The model under review builds one solid part; all positions refer to its coordinate system, in mm. Face numbers are marked on the shaded views. A direction names the side the tool comes from. Give positions to 0.01 mm unless a question says otherwise; leave off trailing zeros. Order: outer loops, then holes, each group sorted by start corner. A loop starts at its lowest first (then second) coordinate and runs counter-clockwise, first axis right, second up. Notation, with made-up numbers: M -34,-15 L -12,-15 A20 cw -12,-4 Z; hole C 15.5,33.25 d9. An arc over 180 degrees is marked long. One line per question, with ' | ' between items. Start each with the question number.
1. Wall thickness on L1, parallel to X at y = -8.2, z = 23.2; L2, parallel to Z at x = -29, y = -7.4; L3, parallel to X at y = -7, z = 22.5: over which ranges is each line inside the solid? List them lowest first.
2. For the marked faces 5, 6, 7 and 8, list the 3-axis set-ups (+Z, -Z, +X, -X, +Y, -Y) from which the entire face can be reached by the end or side of a thin tool; tool diameter is ignored.
3. We need section A-A on x = -29. Write out the cut boundary in (y, z).
4. The part is to be moulded in two halves that separate along X. For the marked faces 1, 2, 3 and 4, say which applies: +X half, -X half, draft (parallel to the pull), parting line (faces both ways), or undercut.
5. We need section C-C on x = -7.5. Write out the cut boundary in (y, z).
6. We need section B-B on z = 10.5. Write out the cut boundary in (x, y).
7. Insertion check: P1, Ø1.3, axis at x = -56.5, y = 4.5, coming from the +Z side; P2, Ø6, axis at x = 21, z = 29, coming from the +Y side; P3, Ø5, axis at y = 5, z = 9.5, coming from the +X side. Each pin has a flat end and moves straight along its axis. Give the tip position at first contact, or say it passes through.
```python
from build123d import *

# Parameters (mm, degrees)
F2_DEPTH     = 9
F3_DEPTH     = 10
F4_R         = 4.1
F4_R_2       = 2.5
F4_R_3       = 1.6
F5_DEPTH     = 24.8
F6_DEPTH     = 3
F4_R_4       = 5
F7_DEPTH     = 6
F4_R_5       = 7.75
F8_DEPTH     = 5
F9_R         = 1.75
F10_DEPTH    = 158.2
F9_R_2       = 3.25
F11_DEPTH    = 2.4
F12_R        = 3.25
F13_DEPTH    = 2.4
F14_R        = 3.4
F14_R_2      = 1.75
F15_DEPTH    = 3
F16_DEPTH    = 25
F17_W        = 100
F17_H        = 9
F18_DEPTH    = 1.1
F20_START    = -1.4
F19_R        = 1.75
F20_DEPTH    = 2.6
F21_DEPTH    = 4.2
F22_W        = 6.7549981495
F22_H        = 2.6
F23_DEPTH    = 4.5
F24_W        = 19
F24_H        = 10
F25_DEPTH    = 16
F26_SIZE     = 5
F27_W        = 19
F27_H        = 10
F28_DEPTH    = 16
F29_SIZE     = 5
F30_R        = 3.15
F31_DEPTH    = 25
F32_R        = 0.4
F33_W        = 87.1225009252
F33_H        = 9
F34_DEPTH    = 4
F35_T1_DEPTH = 9
F37_DEPTH    = 4


# Not quite as in the source:
# - a fillet or chamfer that OpenCascade refuses, or shapes differently, is made with other operations: its cross-section is extruded or revolved along the edge and cut away or added


with BuildPart() as f2:
    # F1 (on face) → F2 (new body)
    with BuildSketch(Plane.XZ):
        Polygon((-55, 28), (-64, 28), (-64, -6), (0, -6), (64, -6), (64, 28), (55, 28), (55, 32.2), (0, 32.2), (-55, 32.2), align=None)
    extrude(amount=F2_DEPTH)

    # F0 (on Front) → F3 (join)
    with BuildSketch(Plane.XZ):
        with BuildLine():
            Line((-57.5, 28), (-64, 28))
            Line((-64, 28), (-64, -6))
            Line((-64, -6), (-43.5, -6))
            Line((-43.5, -6), (-43.5, 0))
            Line((-43.5, 0), (-55, 0))
            ThreePointArc((-55, 0), (-55.3535533906, -0.1464466094), (-55.5, -0.5))
            Line((-55.5, -0.5), (-55.5, -1.5))
            Line((-55.5, -1.5), (-59, -1.5))
            Line((-59, -1.5), (-59, 6.5))
            Line((-59, 6.5), (-54.7, 6.5))
            ThreePointArc((-54.7, 6.5), (-54.3464466094, 6.6464466094), (-54.2, 7))
            Line((-54.2, 7), (-54.2, 13.5))
            ThreePointArc((-54.2, 13.5), (-54.3464466094, 13.8535533906), (-54.7, 14))
            Line((-54.7, 14), (-59, 14))
            Line((-59, 14), (-59, 20.5))
            Line((-59, 20.5), (-57.5, 20.5))
            ThreePointArc((-57.5, 20.5), (-57.1464466094, 20.6464466094), (-57, 21))
            Line((-57, 21), (-57, 27.5))
            ThreePointArc((-57, 27.5), (-57.1464466094, 27.8535533906), (-57.5, 28))
        make_face()
        with BuildLine():
            Line((43.5, -6), (64, -6))
            Line((64, -6), (64, 28))
            Line((64, 28), (57.5, 28))
            ThreePointArc((57.5, 28), (57.1464466094, 27.8535533906), (57, 27.5))
            Line((57, 27.5), (57, 21))
            ThreePointArc((57, 21), (57.1464466094, 20.6464466094), (57.5, 20.5))
            Line((57.5, 20.5), (59, 20.5))
            Line((59, 20.5), (59, 14))
            Line((59, 14), (54.7, 14))
            ThreePointArc((54.7, 14), (54.3464466094, 13.8535533906), (54.2, 13.5))
            Line((54.2, 13.5), (54.2, 7))
            ThreePointArc((54.2, 7), (54.3464466094, 6.6464466094), (54.7, 6.5))
            Line((54.7, 6.5), (59, 6.5))
            Line((59, 6.5), (59, -1.5))
            Line((59, -1.5), (55.5, -1.5))
            Line((55.5, -1.5), (55.5, -0.5))
            ThreePointArc((55.5, -0.5), (55.3535533906, -0.1464466094), (55, 0))
            Line((55, 0), (43.5, 0))
            Line((43.5, 0), (43.5, -6))
        make_face()
    extrude(amount=-F3_DEPTH)

    # F4 (on Front) → F5 (cut)
    with BuildSketch(Plane.XZ):
        with Locations((-29, 23.2)):
            Circle(F4_R)
        with Locations((-45, 23.2)):
            Circle(F4_R)
        with Locations((35.2, 26.5)):
            Circle(F4_R_2)
        with Locations((17.2, 26.5)):
            Circle(F4_R_2)
        with Locations((5.4, 20.2)):
            Circle(F4_R_3)
        with Locations((47, 20.2)):
            Circle(F4_R_3)
    extrude(amount=F5_DEPTH, mode=Mode.SUBTRACT)

    # F4 (on Front) → F6 (cut)
    with BuildSketch(Plane.XZ):
        Polygon((3.7112504626, 17.275), (7.0887495374, 17.275), (8.7774990748, 20.2), (7.0887495374, 23.125), (3.7112504626, 23.125), (2.0225009252, 20.2), align=None)
        with Locations((5.4, 20.2)):
            Circle(F4_R_3, mode=Mode.SUBTRACT)
        Polygon((45.3112504626, 17.275), (48.6887495374, 17.275), (50.3774990748, 20.2), (48.6887495374, 23.125), (45.3112504626, 23.125), (43.6225009252, 20.2), align=None)
        with Locations((47, 20.2)):
            Circle(F4_R_3, mode=Mode.SUBTRACT)
    extrude(amount=F6_DEPTH, mode=Mode.SUBTRACT)

    # F4 (on Front) → F7 (cut)
    with BuildSketch(Plane.XZ):
        with Locations((-45, 23.2)):
            Circle(F4_R_4)
        with Locations((-45, 23.2)):
            Circle(F4_R, mode=Mode.SUBTRACT)
        with Locations((-29, 23.2)):
            Circle(F4_R_4)
        with Locations((-29, 23.2)):
            Circle(F4_R, mode=Mode.SUBTRACT)
    extrude(amount=F7_DEPTH, mode=Mode.SUBTRACT)

    # F4 (on Front) → F8 (cut)
    with BuildSketch(Plane.XZ):
        with Locations((-29, 23.2)):
            Circle(F4_R_5)
        with Locations((-29, 23.2)):
            Circle(F4_R_4, mode=Mode.SUBTRACT)
        with Locations((-45, 23.2)):
            Circle(F4_R_5)
        with Locations((-45, 23.2)):
            Circle(F4_R_4, mode=Mode.SUBTRACT)
    extrude(amount=F8_DEPTH, mode=Mode.SUBTRACT)

    # F9 (on face) → F10 (cut)
    with BuildSketch(Plane(origin=(-64, 0, 0), x_dir=(0, -1, 0), z_dir=(-1, 0, 0))):
        with Locations((-5.2, 24.2)):
            Circle(F9_R)
    extrude(amount=-F10_DEPTH, mode=Mode.SUBTRACT)

    # F9 (on face) → F11 (cut)
    with BuildSketch(Plane(origin=(-64, 0, 0), x_dir=(0, -1, 0), z_dir=(-1, 0, 0))):
        with Locations((-5.2, 24.2)):
            Circle(F9_R_2)
        with Locations((-5.2, 24.2)):
            Circle(F9_R, mode=Mode.SUBTRACT)
    extrude(amount=-F11_DEPTH, mode=Mode.SUBTRACT)

    # F12 (on face) → F13 (cut)
    with BuildSketch(Plane.YZ.offset(64)):
        with Locations((5.2, 24.2)):
            Circle(F12_R)
    extrude(amount=-F13_DEPTH, mode=Mode.SUBTRACT)

    # F14 (on face) → F15 (cut)
    with BuildSketch(Plane(origin=(0, 0, -6), x_dir=(1, 0, 0), z_dir=(0, 0, -1))):
        with Locations((49.8, -5.1)):
            Circle(F14_R)
        with Locations((49.8, -5.1)):
            Circle(F14_R_2, mode=Mode.SUBTRACT)
        with Locations((-48.5, -5.1)):
            Circle(F14_R)
        with Locations((-48.5, -5.1)):
            Circle(F14_R_2, mode=Mode.SUBTRACT)
        with Locations((49.8, -5.1)):
            Circle(F14_R_2)
    extrude(amount=-F15_DEPTH, mode=Mode.SUBTRACT)

    # F14 (on face) → F16 (cut)
    with BuildSketch(Plane(origin=(0, 0, -6), x_dir=(1, 0, 0), z_dir=(0, 0, -1))):
        with Locations((49.8, -5.1)):
            Circle(F14_R_2)
        with Locations((-48.5, -5.1)):
            Circle(F14_R_2)
    extrude(amount=-F16_DEPTH, mode=Mode.SUBTRACT)

    # F17 (on face) → F18 (join)
    with BuildSketch(Plane.XY.offset(32.2)):
        with Locations((5, -4.5)):
            Rectangle(F17_W, F17_H)
    extrude(amount=F18_DEPTH)

    # F19 (on face) → F20 (cut)
    with BuildSketch(Plane.XY.offset(33.3).offset(F20_START)):
        Polygon((35.3112504626, -7.425), (38.6887495374, -7.425), (40.3774990748, -4.5), (38.6887495374, -1.575), (35.3112504626, -1.575), (33.6225009252, -4.5), align=None)
        with Locations((37, -4.5)):
            Circle(F19_R, mode=Mode.SUBTRACT)
        Polygon((-38.6887495374, -7.425), (-35.3112504626, -7.425), (-33.6225009252, -4.5), (-35.3112504626, -1.575), (-38.6887495374, -1.575), (-40.3774990748, -4.5), align=None)
        with Locations((-37, -4.5)):
            Circle(F19_R, mode=Mode.SUBTRACT)
    extrude(amount=-F20_DEPTH, mode=Mode.SUBTRACT)

    # F19 (on face) → F21 (cut)
    with BuildSketch(Plane.XY.offset(33.3)):
        with Locations((-37, -4.5)):
            Circle(F19_R)
        with Locations((37, -4.5)):
            Circle(F19_R)
    extrude(amount=-F21_DEPTH, mode=Mode.SUBTRACT)

    # F22 (on face) → F23 (cut)
    with BuildSketch(Plane(origin=(0, 0, 0), x_dir=(-1, 0, 0), z_dir=(0, 1, 0))):
        with Locations((-37, 30.6)):
            Rectangle(F22_W, F22_H)
        with Locations((37, 30.6)):
            Rectangle(F22_W, F22_H)
    extrude(amount=-F23_DEPTH, mode=Mode.SUBTRACT)

    # F24 (on face) → F25 (join)
    with BuildSketch(Plane(origin=(-64, 0, 0), x_dir=(0, -1, 0), z_dir=(-1, 0, 0))):
        with Locations((-0.5, -1)):
            Rectangle(F24_W, F24_H)
    extrude(amount=F25_DEPTH)

    # F26
    f26_edges = [f2.edges().sort_by_distance(p)[0] for p in [
        (-80, -9, -1),
        (-80, 10, -1),
    ]]
    chamfer(f26_edges, length=F26_SIZE)

    # F27 (on face) → F28 (join)
    with BuildSketch(Plane.YZ.offset(64)):
        with Locations((0.5, -1)):
            Rectangle(F27_W, F27_H)
    extrude(amount=F28_DEPTH)

    # F29
    f29_edges = [f2.edges().sort_by_distance(p)[0] for p in [
        (80, 10, -1),
        (80, -9, -1),
    ]]
    chamfer(f29_edges, length=F29_SIZE)

    # F30 (on face) → F31 (cut)
    with BuildSketch(Plane(origin=(0, 0, -6), x_dir=(1, 0, 0), z_dir=(0, 0, -1))):
        with Locations((-73, -0.5)):
            Circle(F30_R)
        with Locations((73, -0.5)):
            Circle(F30_R)
    extrude(amount=-F31_DEPTH, mode=Mode.SUBTRACT)

    # F32
    f32_edges = [f2.edges().sort_by_distance(p)[0] for p in [
        (64, 0.5, 28),
        (55, -4.5, 33.3),
        (-64, 0.5, 28),
        (-55, -4.5, 28),
        (-55, -4.5, 32.2),
        (-45, -4.5, 32.2),
        (-45, -4.5, 33.3),
        (-64, 0.5, 4),
        (64, 0.5, 4),
    ]]
    fillet(f32_edges, radius=F32_R)

    # F33 (on face) → F34 (cut)
    with BuildSketch(Plane(origin=(0, 0, -6), x_dir=(1, 0, 0), z_dir=(0, 0, -1))):
        with Locations((0.0612504626, 4.5)):
            Rectangle(F33_W, F33_H)
    extrude(amount=-F34_DEPTH, mode=Mode.SUBTRACT)

    # F35: fillet of radius 3 on 2 edges, made by hand

    # F35_s2 → F35_t1 (join)
    with BuildSketch(Plane.XZ):
        with BuildLine():
            ThreePointArc((-43.5, -5), (-42.6213203436, -2.8786796564), (-40.5, -2))
            Line((-40.5, -2), (-43.5, -2))
            Line((-43.5, -2), (-43.5, -5))
        make_face()
        with BuildLine():
            ThreePointArc((40.6225009252, -2), (42.7438212688, -2.8786796564), (43.6225009252, -5))
            Line((43.6225009252, -5), (43.6225009252, -2))
            Line((43.6225009252, -2), (40.6225009252, -2))
        make_face()
    extrude(amount=F35_T1_DEPTH)

    # F36 (on face) → F37 (cut)
    with BuildSketch(Plane(origin=(0, 0, 0), x_dir=(-1, 0, 0), z_dir=(0, 1, 0))):
        with BuildLine():
            Line((22.4636435891, 27.3639578372), (19.415192306, 27.3639578372))
            Line((19.415192306, 27.3639578372), (19.415192306, 19.0618205816))
            Line((19.415192306, 19.0618205816), (22.4472928418, 19.0618205816))
            ThreePointArc((22.4472928418, 19.0618205816), (21.5553381381, 21.0460478738), (21.25, 23.2))
            ThreePointArc((21.25, 23.2), (21.5595946957, 25.3686099022), (22.4636435891, 27.3639578372))
        make_face()
        with BuildLine():
            Line((38.4636435891, 27.3639578372), (35.5363564109, 27.3639578372))
            ThreePointArc((35.5363564109, 27.3639578372), (36.7499849698, 23.2152633041), (35.5527071582, 19.0618205816))
            Line((35.5527071582, 19.0618205816), (38.4472928418, 19.0618205816))
            ThreePointArc((38.4472928418, 19.0618205816), (37.5553381381, 21.0460478738), (37.25, 23.2))
            ThreePointArc((37.25, 23.2), (37.5595946957, 25.3686099022), (38.4636435891, 27.3639578372))
        make_face()
        with BuildLine():
            Line((53.6553673446, 27.3639578372), (51.5363564109, 27.3639578372))
            ThreePointArc((51.5363564109, 27.3639578372), (52.7499849698, 23.2152633041), (51.5527071582, 19.0618205816))
            Line((51.5527071582, 19.0618205816), (53.6553673446, 19.0618205816))
            Line((53.6553673446, 19.0618205816), (53.6553673446, 27.3639578372))
        make_face()
    extrude(amount=-F37_DEPTH, mode=Mode.SUBTRACT)


solid = f2.part
```
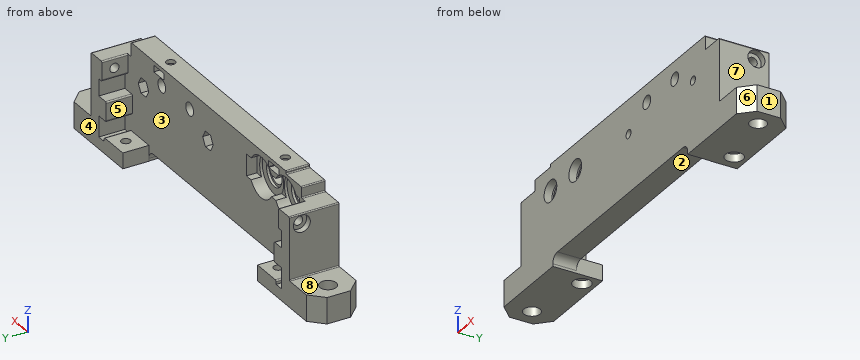
Entries:
1) L1: x = -64 to -49.1, -40.9 to -33.1, -24.9 to 64 | L2: z = -2 to 19.1, 27.3 to 33.3 | L3: x = -64 to -49.04, -40.96 to -33.04, -24.96 to 64
2) face 5: +Z, +Y | face 6: +Z, -Z, +X, -Y | face 7: +Z, +X, +Y, -Y | face 8: +Z, -X, +Y, -Y
3) outline: M -9,-2 L 0,-2 L 0,15.45 L -5,15.45 L -5,18.2 L -6,18.2 L -6,19.1 L -9,19.1 Z; M -9,27.3 L -6,27.3 L -6,28.2 L -5,28.2 L -5,30.95 L 0,30.95 L 0,33.3 L -9,33.3 Z
4) face 1: +X half | face 2: undercut | face 3: undercut | face 4: draft
5) outline: M -9,-2 L 0,-2 L 0,33.3 L -9,33.3 Z
6) outline: M -64,-9 L 64,-9 L 64,10 L 54.2,10 L 54.2,0 L -54.2,0 L -54.2,10 L -64,10 Z
7) P1: stops at z = 27.86 | P2: stops at y = 0 | P3: stops at x = 64
